Autodesk Inventor part; units mm, degrees
ref_plane "YZ Plane" through (0, 0, 0) normal (1, 0, 0) x (0, 1, 0)
ref_plane "XZ Plane" through (0, 0, 0) normal (0, 1, 0) x (-1, 0, 0)
ref_plane "XY Plane" through (0, 0, 0) normal (0, 0, 1) x (1, 0, 0)
sketch "Sketch1" plane through (0, 0, 0) normal (0, 0, 1) x (1, 0, 0)
  circle A0 centre (0, 0) radius 20
  dimension "d0" = 40
extrude "Extrusion1" add sketch "Sketch1" along normal blind 120
sketch "Sketch2" plane through (0, 0, 0) normal (0, 0, -1) x (-1, 0, 0)
  point P0 (0, 0)
  point P1 (0, 0)
hole "Hole1" at (0, 0, 0) at (0, 0, 0) direction (0, 0, 1) diameter 35 depth 86.25
shell "Shell1" thickness 1.5 removed faces 1 at (-2.364, 6.2334, 120)
sketch "Sketch3" plane through (0, 0, 87.75) normal (0, 0, 1) x (1, 0, 0)
  point P0 (0, 0)
  point P1 (-0.8402, 0.3734)
hole "Hole2" at (-0.8402, 0.3734, 87.75) direction (0, 0, -1) diameter 10 depth 86.25
fillet "Fillet1" radius 2 1 edges at (-18.5, 0, 120)
thread "Thread1"
thread "Thread2"
properties part number "badan lampu" material "Aluminum 6061-AHC"
The listing builds one solid part. Answer for the finished solid, in the listing's coordinates (mm). A direction names the side the tool comes from. Coordinates: 2 decimals unless noted, no trailing zeros. Order: outer loops, then holes, each group sorted by start corner. A loop starts at its lowest first (then second) coordinate and runs counter-clockwise, first axis right, second up. Notation, with made-up numbers: (-37, -5) -> (-23, -5) arc R19 ccw to (-23, -1) -> close; hole circle Ø1 at (-18.75, 74). An arc over 180 degrees is marked (long way). Answer in a Markdown table with one row per item. Add a question column.
Item 1: Find section B-B (z = 111). Write down the section's boundary in (x, y), then the cut area to 3 significant figures.
Item 2: Each of these flat-tipped pins is pushed along its axis until it touches: P1, Ø13, axis at x = -0.84, y = 0.37, coming from the -Z side; P2, Ø1, axis at y = 5.5, z = 30.5, coming from the -X side; P3, Ø12, axis at x = 10.5, y = -3, coming from the +Z side; P4, Ø4, axis at x = 13, y = -12, coming from the -Z side. Where does it stop, or does it pass through?
Item 3: Find the intervals of material crossed by L1, parallel to Y at x = 0, z = 107.5; L2, parallel to Z at x = -9.5, y = -6; L3, parallel to X at y = -10, z = 30, in increasing order. Write a range as from..to.
Item 4: Find section A-A (z = 73). Write down the section's boundary in (x, y).
Item 5: Determine the mould class of faces 1 (the face through (-4.336, 19.524, 59.16)), 2 (the face through (-4.01, 18.06, 102.69)), 3 (the face through (0, -18, 0)) for opening direction X: +X half, -X half, draft (parallel to the pull), parting line (faces both ways), or undercut.
Item 6: Which of the six approach directions +Z, -Z, +X, -X, +Y, -Y give full straight-line access (tool end or side, diameter ignored) to faces 4 (the face through (4, 4, 87.75)), 5 (the face through (4, 4, 86.25)), 6 (the face through (4.04, 1.46, 86.99))?
Result set:
| question | item | result |
|---|---|---|
| 1 | outline | circle Ø40 at (0, 0); hole circle Ø37 at (0, 0) |
| 1 | area | 181 mm² |
| 2 | P1 | stops at z = 86.25 |
| 2 | P2 | stops at x = -19.36 |
| 2 | P3 | stops at z = 87.75 |
| 2 | P4 | stops at z = 0 |
| 3 | L1 | y = -20..-18.5, 18.5..20 |
| 3 | L2 | z = 86.25..87.75 |
| 3 | L3 | x = -17.32..-14.36, 14.36..17.32 |
| 4 | outline | circle Ø40 at (0, 0); hole circle Ø35 at (0, 0) |
| 5 | face 1 | parting line |
| 5 | face 2 | undercut |
| 5 | face 3 | draft |
| 6 | face 4 | +Z |
| 6 | face 5 | -Z |
| 6 | face 6 | +Z, -Z |
